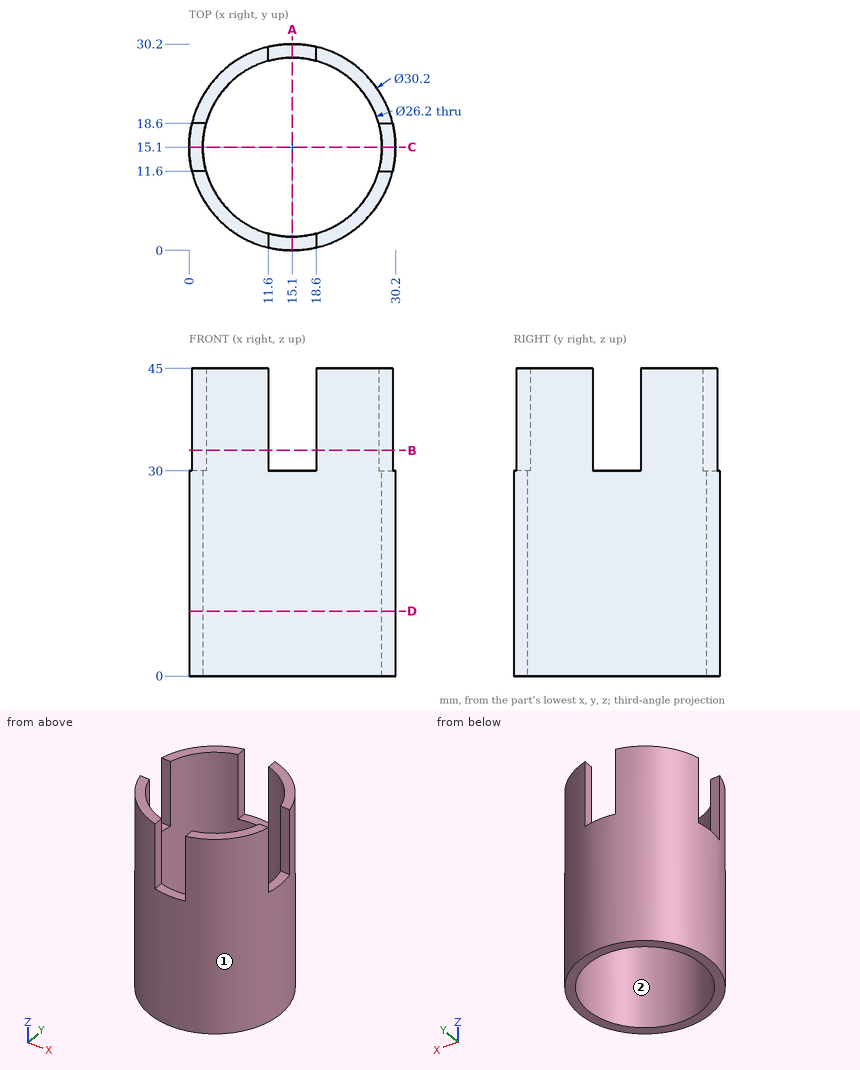
Geometry: see drawing. Coordinates: mm, zero at the bounding-box minimum. Give positions to 0.01 mm unless a question says otherwise; leave off trailing zeros. Loops run counter-clockwise (first coordinate to the right, second up) from the corner with the lowest first, then second, coordinate; pieces in that order, holes last. Notation, with made-up numbers: (45, 65.25) -> (104, 65.25) arc R8 ccw to (104, 69.25) -> close; hole circle Ø1 at (80, -34). An arc over 180 degrees is marked (long way). Answer as a JSON object with one key per item and string values. Group by question number.
Item 1: Pull-direction query (Y, two-part tool) for the marked faces 1 and 2; classes: released by +Y, released by -Y, zero draft, split by the parting line, or undercut.
Item 2: Cut plane A-A, the plane x = 15.1. Return the cut outline in (y, z), and give its area (3 significant figures).
Item 3: Cut plane D-D, the plane z = 9.5. Return the cut outline in (x, y).
Item 4: Line query: probe 1 along X at (y, z) = (15, 10); probe 2 along X at (y, z) = (23.5, 23). Output: solid intervals per line, ascending.
Item 5: Pin query (flat end, axial travel): P1, Ø0.7, axis at x = 14.5, y = 1.5, coming from the +Z side; P2, Ø10, axis at y = 5, z = 35.5, coming from the +X side; P3, Ø10, axis at x = 8.5, z = 28, coming from the +Y side (3 decimals); P4, Ø3, axis at y = 14.5, z = 33, coming from the +X side. Return the tip coordinate at first contact, or that it passes through.
Item 6: Cut plane B-B, the plane z = 33. Return the cut outline in (x, y), and give its area (3 significant figures).
Checks:
{
 "1": {"face 1": "split by the parting line", "face 2": "undercut"},
 "2": {"outline": "(0, 0) -> (2, 0) -> (2, 30) -> (0, 30) -> close; (28.2, 0) -> (30.2, 0) -> (30.2, 30) -> (28.2, 30) -> close", "area": "120 mm²"},
 "3": {"outline": "circle Ø30.2 at (15.1, 15.1); hole circle Ø26.2 at (15.1, 15.1)"},
 "4": {"probe 1": "x = 0 to 2, 28.2 to 30.2", "probe 2": "x = 2.55 to 5.05, 25.15 to 27.65"},
 "5": {"P1": "stops at z = 30", "P2": "stops at x = 29.31", "P3": "stops at y = 30.115", "P4": "passes through"},
 "6": {"outline": "(0.41, 11.6) arc R15.1 ccw to (11.6, 0.41) -> (11.6, 2.48) arc R13.1 cw to (2.48, 11.6) -> close; (0.41, 18.6) -> (2.48, 18.6) arc R13.1 cw to (11.6, 27.72) -> (11.6, 29.79) arc R15.1 ccw to start; (18.6, 0.41) arc R15.1 ccw to (29.79, 11.6) -> (27.72, 11.6) arc R13.1 cw to (18.6, 2.48) -> close; (18.6, 27.72) arc R13.1 cw to (27.72, 18.6) -> (29.79, 18.6) arc R15.1 ccw to (18.6, 29.79) -> close", "area": "121 mm²"}
}
